```python
from build123d import *

# Parameters (mm, degrees)
F1_DEPTH = 4.4958


with BuildPart() as f1:
    # F0 (on Top) → F1 (new body)
    with BuildSketch(Plane.XY):
        Polygon((50.8, 50.8), (-50.8, 50.8), (-55.2958, 50.8), (-55.2958, 38.1), (-50.8, 38.1), (-50.8, 26.8478), (-48.26, 26.8478), (-48.26, 28.6385), (-45.75175, 28.6385), (-45.75175, 26.8478), (-42.3418, 26.8478), (-42.3418, 23.9522), (-45.75175, 23.9522), (-45.75175, 22.1615), (-48.26, 22.1615), (-48.26, 23.9522), (-50.8, 23.9522), (-50.8, 12.7), (-55.2958, 12.7), (-55.2958, 0), (-55.2958, -12.7), (-50.8, -12.7), (-50.8, -23.9522), (-48.26, -23.9522), (-48.26, -22.1615), (-45.75175, -22.1615), (-45.75175, -23.9522), (-42.3418, -23.9522), (-42.3418, -26.8478), (-45.75175, -26.8478), (-45.75175, -28.6385), (-48.26, -28.6385), (-48.26, -26.8478), (-50.8, -26.8478), (-50.8, -38.1), (-55.2958, -38.1), (-55.2958, -50.8), (-50.8, -50.8), (50.8, -50.8), (55.2958, -50.8), (55.2958, -38.1), (50.8, -38.1), (50.8, -26.8478), (48.26, -26.8478), (48.26, -28.6385), (45.75175, -28.6385), (45.75175, -26.8478), (42.3418, -26.8478), (42.3418, -23.9522), (45.75175, -23.9522), (45.75175, -22.1615), (48.26, -22.1615), (48.26, -23.9522), (50.8, -23.9522), (50.8, -12.7), (55.2958, -12.7), (55.2958, 0), (55.2958, 12.7), (50.8, 12.7), (50.8, 23.9522), (48.26, 23.9522), (48.26, 22.1615), (45.75175, 22.1615), (45.75175, 23.9522), (42.3418, 23.9522), (42.3418, 26.8478), (45.75175, 26.8478), (45.75175, 28.6385), (48.26, 28.6385), (48.26, 26.8478), (50.8, 26.8478), (50.8, 38.1), (55.2958, 38.1), (55.2958, 50.8), align=None)
    extrude(amount=F1_DEPTH)


solid = f1.part
```
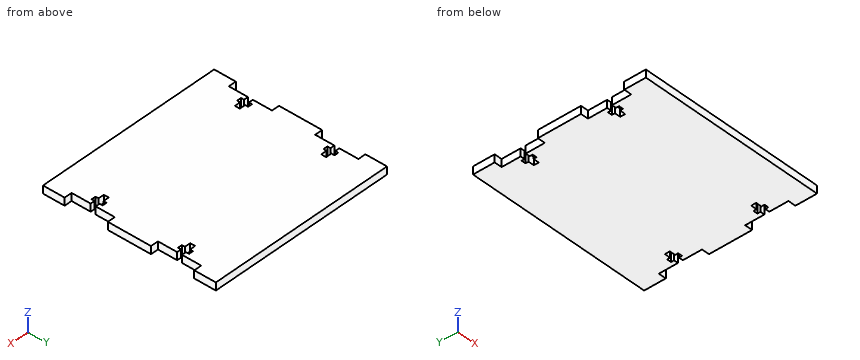
Verification items for the finished model (mm, model axes). Round coordinates to 2 decimals unless told otherwise and drop trailing zeros. Write each loop counter-clockwise with the first axis right and the second up, starting at its lowest first coordinate (ties: lowest second). Pieces come first, ordered by that corner, then holes.
1. Scan lines: L1, parallel to Y at x = 50, z = 1.45; L2, parallel to X at y = 23, z = 2.95; L3, parallel to Y at x = -46, z = 2.9. Record each from-to range of solid material in increasing order.
2. Section check B-B on y = 33.5. Enter the section's corners in (x, z).
3. Gauge pin test, flat ends, axial feed: P1, Ø2, axis at y = 23.5, z = 1, coming from the +X side; P2, Ø0.9, axis at y = 27.5, z = 1.5, coming from the -X side; P3, Ø1.4, axis at y = -25, z = 2.5, coming from the -X side. Record the tip position at first contact, or that the pin passes through.
4. Section check A-A on x = 44. Enter the section's corners in (y, z), plus the area to 3 significant figures.
Answer:
1. L1: y = -50.8 to -26.85, -23.95 to 23.95, 26.85 to 50.8
1. L2: x = -50.8 to -48.26, -45.75 to 45.75, 48.26 to 50.8
1. L3: y = -50.8 to -28.64, -22.16 to 22.16, 28.64 to 50.8
2. outline: (-50.8, 0) - (50.8, 0) - (50.8, 4.5) - (-50.8, 4.5) - close
3. P1: stops at x = 50.8
3. P2: stops at x = -50.8
3. P3: stops at x = -42.34
4. outline: (-50.8, 0) - (-26.85, 0) - (-26.85, 4.5) - (-50.8, 4.5) - close; (-23.95, 0) - (23.95, 0) - (23.95, 4.5) - (-23.95, 4.5) - close; (26.85, 0) - (50.8, 0) - (50.8, 4.5) - (26.85, 4.5) - close
4. area: 431 mm2
